CAD build for the part. Positions are in the model's coordinates, mm. Face numbers are marked on the shaded views. A direction names the side the tool comes from. Coordinates: 2 decimals unless noted, no trailing zeros. Loops run counter-clockwise (first coordinate to the right, second up) from the corner with the lowest first, then second, coordinate; pieces in that order, holes last. Notation, with made-up numbers: (-12.75, -26) -> (20.25, -26) arc R8 ccw to (20.25, -14) -> close; hole circle Ø3 at (54.25, 28). An arc over 180 degrees is marked (long way). Answer as a JSON object with one key per item and string values. Group by question number.
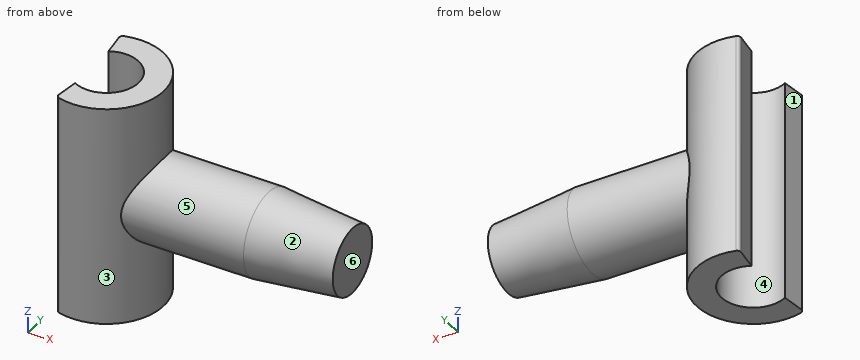
from build123d import *

# Parameters (mm, degrees)
F2_R     = 7.5
F3_DEPTH = 40
F4_SIZE2 = 15.1
F4_SIZE  = 1.5
F5_DEPTH = 2.5
F6_DEPTH = 20


with BuildPart() as f3:
    # F2 (on offset) → F3 (new body)
    with BuildSketch(Plane.YZ.offset(4)):
        Circle(F2_R)
    extrude(amount=F3_DEPTH)

    # F4
    f4_edges = [f3.edges().sort_by_distance(p)[0] for p in [
        (44, -7.5, 0),
    ]]
    f4_side = f3.faces().sort_by_distance((44, 0, 0))[0]
    chamfer(f4_edges, length=F4_SIZE, length2=F4_SIZE2, reference=f4_side)

    # F2 (on offset) → F5 (cut)
    with BuildSketch(Plane.YZ.offset(4)):
        Circle(F2_R)
    extrude(amount=F5_DEPTH, mode=Mode.SUBTRACT)

    # F0 (on Top) → F6 (join, symmetric)
    with BuildSketch(Plane.XY):
        with BuildLine():
            ThreePointArc((-3.2107160512, -9.1318440865), (-3.1021542498, -9.6020282515), (-2.711222774, -9.8849264575))
            ThreePointArc((-2.711222774, -9.8849264575), (10.25, 0), (-2.711222774, 9.8849264575))
            ThreePointArc((-2.711222774, 9.8849264575), (-3.1021542498, 9.6020282515), (-3.2107160512, 9.1318440865))
            Line((-3.2107160512, 9.1318440865), (-2.6748366384, 5.089965529))
            ThreePointArc((-2.6748366384, 5.089965529), (5.7500000112, 0), (-2.6748366384, -5.089965529))
            Line((-2.6748366384, -5.089965529), (-3.2107160512, -9.1318440865))
        make_face()
    extrude(amount=F6_DEPTH, both=True)


solid = f3.part
Item 1: Pull direction X, two halves, no side cores. Call the marked faces 1, 2, 3 and 4: +X half, -X half, draft (parallel to the pull), parting line (faces both ways), or undercut.
Item 2: Drill centre lines: L1, parallel to Y at x = 0, z = -4; L2, parallel to Z at x = 13, y = 0; L3, parallel to Y at x = 14, z = 4.5. Where is each one in solid material? Low to high.
Item 3: Band-saw the part on A-A, the plane x = 0. List the corners of the cut face in (y, z).
Item 4: Band-saw the part on B-B, the plane z = 0. List the corners of the cut face in (x, y), and give its area (3 significant figures).
Item 5: Band-saw the part on D-D, the plane x = 22.5. List the corners of the cut face in (y, z), and give its area (3 significant figures).
Item 6: Flat gauge pins, fed straight in: P1, Ø2, axis at x = 20, z = -1.5, coming from the -Y side; P2, Ø5, axis at x = 7, z = 10, coming from the +Y side; P3, Ø6, axis at x = 8, y = -7, coming from the -Z side; P4, Ø6, axis at x = 38.5, z = -8, coming from the -Y side. Where does each tip first touch, or does it go through?
Item 7: Band-saw the part on C-C, the plane y = 0. List the corners of the cut face in (x, z), and give its area (3 significant figures).
Item 8: 3-axis set-ups, long thin cutter, end or side, ignore diameter. For the marked faces 5 and 6: which of +Z, -Z, +X, -X, +Y, -Y reach the whole face in a straight line?
Reply:
{
 "1": {"face 1": "-X half", "face 2": "+X half", "face 3": "parting line", "face 4": "undercut"},
 "2": {"L1": "-10.25 to -5.75, 5.75 to 10.25", "L2": "-7.5 to 7.5", "L3": "-6 to 6"},
 "3": {"outline": "(-10.25, -20) -> (-5.75, -20) -> (-5.75, 20) -> (-10.25, 20) -> close; (5.75, -20) -> (10.25, -20) -> (10.25, 20) -> (5.75, 20) -> close"},
 "4": {"outline": "(-3.21, -9.13) arc R0.69 ccw to (-2.71, -9.88) arc R10.25 ccw to (6.99, -7.5) -> (28.9, -7.5) -> (44, -6) -> (44, 6) -> (28.9, 7.5) -> (6.99, 7.5) arc R10.25 ccw to (-2.71, 9.88) arc R0.69 ccw to (-3.21, 9.13) -> (-2.67, 5.09) arc R5.75 cw (long way) to (-2.67, -5.09) -> close", "area": "639 mm²"},
 "5": {"outline": "circle Ø15 at (0, 0)", "area": "177 mm²"},
 "6": {"P1": "y = -7.48", "P2": "y = 9.21", "P3": "z = -20", "P4": "y = -4.26"},
 "7": {"outline": "(5.75, -20) -> (10.25, -20) -> (10.25, -7.5) -> (28.9, -7.5) -> (44, -6) -> (44, 6) -> (28.9, 7.5) -> (10.25, 7.5) -> (10.25, 20) -> (5.75, 20) -> close", "area": "664 mm²"},
 "8": {"face 5": "+X", "face 6": "+Z, -Z, +X, +Y, -Y"}
}
